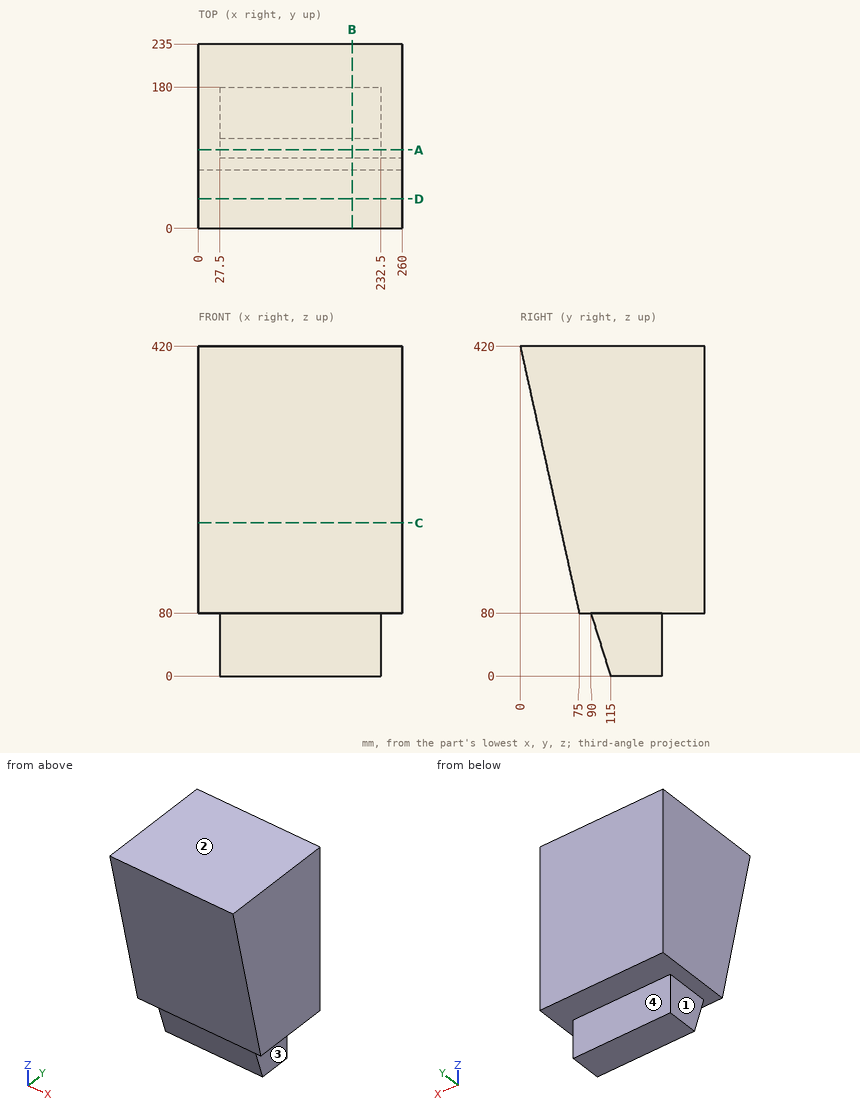
The drawing under review shows one solid part. Ordinate dimensions are in mm from its lowest x, y, z. A direction names the side the tool comes from. Coordinates: 2 decimals unless noted, no trailing zeros. Write each loop counter-clockwise with the first axis right and the second up, starting at its lowest first coordinate (ties: lowest second). Pieces come first, ordered by that corner, then holes.
1) Insertion check: pin 1 (3 mm diameter, centred on x = 56, y = 125.5, fed in from -Z); pin 2 (1 mm diameter, centred on x = 48.5, z = 181.5, fed in from -Y); pin 3 (24 mm diameter, centred on x = 128.5, z = 47.5, fed in from +Y). Each pin has a flat end and moves straight along its axis. Give the tip position at first contact, or say it passes through.
2) To check wall thickness, follow L1, parallel to Z at x = 17.5, y = 128.5; L2, parallel to Y at x = 121, z = 374.5; L3, parallel to Y at x = 64.5, z = 335. State the ranges of each line that lie inside material, in increasing order.
3) Machinability: for the marked faces 1, 2, 3 and 4, which of the approach directions +Z, -Z, +X, -X, +Y, -Y give a long, thin tool a straight path to every point of the face, cutting with its end or side? Answer none if there is none.
4) Add section B-B (x = 196). Write out the cut boundary in (y, z).
5) Add section A-A (y = 100). Write out the cut boundary in (x, z).
6) Add section D-D (y = 37.5). Write out the cut boundary in (x, z).
7) Add section C-C (z = 195). Write out the cut boundary in (x, y).
Check result:
1. pin 1: stops at z = 0
1. pin 2: stops at y = 52.5
1. pin 3: stops at y = 180
2. L1: z = 80 to 420
2. L2: y = 10.04 to 235
2. L3: y = 18.75 to 235
3. face 1: -Z, -X, +Y, -Y
3. face 2: +Z, +X, -X, +Y, -Y
3. face 3: -Z, +X, +Y, -Y
3. face 4: -Z, +X, -X, +Y
4. outline: (0, 420) - (75, 80) - (90, 80) - (115, 0) - (180, 0) - (180, 80) - (235, 80) - (235, 420) - close
5. outline: (0, 80) - (27.5, 80) - (27.5, 48) - (232.5, 48) - (232.5, 80) - (260, 80) - (260, 420) - (0, 420) - close
6. outline: (0, 250) - (260, 250) - (260, 420) - (0, 420) - close
7. outline: (0, 49.63) - (260, 49.63) - (260, 235) - (0, 235) - close
